from build123d import *

# Parameters (mm, degrees)
SKETCH097_R   = 2.6035
EXTRUDE_DEPTH = 195.262


with BuildPart() as part:
    # Sketch097 → Extrude (new body)
    with BuildSketch(Plane.XY):
        with BuildLine():
            ThreePointArc((12.7, 6.333084), (12.192, 5.825084), (12.7, 5.317084))
            Line((12.7, 4.287469), (12.7, 5.317084))
            ThreePointArc((11.650988, 3.238457), (12.392751, 3.545706), (12.7, 4.287469))
            Line((11.539212, 3.238457), (11.650988, 3.238457))
            ThreePointArc((10.4902, 4.287469), (10.797449, 3.545706), (11.539212, 3.238457))
            Line((10.4902, 6.402089), (10.4902, 4.287469))
            ThreePointArc((10.4902, 6.402089), (9.856505, 7.351068), (8.737131, 7.129409))
            Line((5.441006, 3.840816), (8.737131, 7.129409))
            ThreePointArc((5.441006, 3.840816), (4.750878, 2.809883), (4.5085, 1.593186))
            Line((4.5085, -1.593186), (4.5085, 1.593186))
            ThreePointArc((4.5085, -1.593186), (4.750878, -2.809883), (5.441006, -3.840816))
            Line((8.737131, -7.129409), (5.441006, -3.840816))
            ThreePointArc((8.737131, -7.129409), (9.856505, -7.351068), (10.4902, -6.402089))
            Line((10.4902, -4.287469), (10.4902, -6.402089))
            ThreePointArc((11.539212, -3.238457), (10.797449, -3.545706), (10.4902, -4.287469))
            Line((11.650988, -3.238457), (11.539212, -3.238457))
            ThreePointArc((12.7, -4.287469), (12.392751, -3.545706), (11.650988, -3.238457))
            Line((12.7, -5.317084), (12.7, -4.287469))
            ThreePointArc((12.7, -5.317084), (12.192, -5.825084), (12.7, -6.333084))
            Line((12.7, -9.5504), (12.7, -6.333084))
            ThreePointArc((12.7, -9.5504), (12.192, -10.058323), (12.699847, -10.5664))
            ThreePointArc((10.566443, -12.699848), (12.082538, -12.082507), (12.699847, -10.5664))
            ThreePointArc((10.566443, -12.699848), (10.058367, -12.192), (9.550443, -12.7))
            Line((6.333127, -12.7), (9.550443, -12.7))
            ThreePointArc((6.333127, -12.7), (5.825127, -12.192), (5.317127, -12.7))
            Line((4.287512, -12.7), (5.317127, -12.7))
            ThreePointArc((3.2385, -11.650988), (3.545749, -12.392751), (4.287512, -12.7))
            Line((3.2385, -11.539212), (3.2385, -11.650988))
            ThreePointArc((4.287512, -10.4902), (3.545749, -10.797449), (3.2385, -11.539212))
            Line((6.416408, -10.4902), (4.287512, -10.4902))
            ThreePointArc((6.416408, -10.4902), (7.414731, -9.822813), (7.17965, -8.645193))
            Line((3.95227, -5.42369), (7.17965, -8.645193))
            ThreePointArc((3.95227, -5.42369), (2.922936, -4.736929), (1.709254, -4.4958))
            Line((-1.709254, -4.4958), (1.709254, -4.4958))
            ThreePointArc((-1.709254, -4.4958), (-2.922936, -4.736929), (-3.95227, -5.42369))
            Line((-7.17965, -8.645193), (-3.95227, -5.42369))
            ThreePointArc((-7.17965, -8.645193), (-7.414731, -9.822813), (-6.416408, -10.4902))
            Line((-4.287512, -10.4902), (-6.416408, -10.4902))
            ThreePointArc((-3.2385, -11.539212), (-3.545749, -10.797449), (-4.287512, -10.4902))
            Line((-3.2385, -11.650988), (-3.2385, -11.539212))
            ThreePointArc((-4.287512, -12.7), (-3.545749, -12.392751), (-3.2385, -11.650988))
            Line((-5.317127, -12.7), (-4.287512, -12.7))
            ThreePointArc((-5.317127, -12.7), (-5.825127, -12.192), (-6.333127, -12.7))
            Line((-9.550443, -12.7), (-6.333127, -12.7))
            ThreePointArc((-9.550443, -12.7), (-10.058367, -12.192), (-10.566443, -12.699848))
            ThreePointArc((-12.699847, -10.5664), (-12.082538, -12.082507), (-10.566443, -12.699848))
            ThreePointArc((-12.699847, -10.5664), (-12.192, -10.058323), (-12.7, -9.5504))
            Line((-12.7, -6.333084), (-12.7, -9.5504))
            ThreePointArc((-12.7, -6.333084), (-12.192, -5.825084), (-12.7, -5.317084))
            Line((-12.7, -4.287469), (-12.7, -5.317084))
            ThreePointArc((-11.650988, -3.238457), (-12.392751, -3.545706), (-12.7, -4.287469))
            Line((-11.539212, -3.238457), (-11.650988, -3.238457))
            ThreePointArc((-10.4902, -4.287469), (-10.797449, -3.545706), (-11.539212, -3.238457))
            Line((-10.4902, -6.402089), (-10.4902, -4.287469))
            ThreePointArc((-10.4902, -6.402089), (-9.856505, -7.351068), (-8.737131, -7.129409))
            Line((-5.441006, -3.840816), (-8.737131, -7.129409))
            ThreePointArc((-5.441006, -3.840816), (-4.750878, -2.809883), (-4.5085, -1.593186))
            Line((-4.5085, 1.593186), (-4.5085, -1.593186))
            ThreePointArc((-4.5085, 1.593186), (-4.750878, 2.809883), (-5.441006, 3.840816))
            Line((-8.737131, 7.129409), (-5.441006, 3.840816))
            ThreePointArc((-8.737131, 7.129409), (-9.856505, 7.351068), (-10.4902, 6.402089))
            Line((-10.4902, 4.287469), (-10.4902, 6.402089))
            ThreePointArc((-11.539212, 3.238457), (-10.797449, 3.545706), (-10.4902, 4.287469))
            Line((-11.650988, 3.238457), (-11.539212, 3.238457))
            ThreePointArc((-12.7, 4.287469), (-12.392751, 3.545706), (-11.650988, 3.238457))
            Line((-12.7, 5.317084), (-12.7, 4.287469))
            ThreePointArc((-12.7, 5.317084), (-12.192, 5.825084), (-12.7, 6.333084))
            Line((-12.7, 9.5504), (-12.7, 6.333084))
            ThreePointArc((-12.7, 9.5504), (-12.192, 10.058323), (-12.699847, 10.5664))
            ThreePointArc((-10.566443, 12.699848), (-12.082538, 12.082507), (-12.699847, 10.5664))
            ThreePointArc((-10.566443, 12.699848), (-10.058367, 12.192), (-9.550443, 12.7))
            Line((-6.333127, 12.7), (-9.550443, 12.7))
            ThreePointArc((-6.333127, 12.7), (-5.825127, 12.192), (-5.317127, 12.7))
            Line((-4.287512, 12.7), (-5.317127, 12.7))
            ThreePointArc((-3.2385, 11.650988), (-3.545749, 12.392751), (-4.287512, 12.7))
            Line((-3.2385, 11.539212), (-3.2385, 11.650988))
            ThreePointArc((-4.287512, 10.4902), (-3.545749, 10.797449), (-3.2385, 11.539212))
            Line((-6.476789, 10.4902), (-4.287512, 10.4902))
            ThreePointArc((-6.476789, 10.4902), (-7.432222, 9.851404), (-7.207036, 8.724371))
            Line((-3.898273, 5.423169), (-7.207036, 8.724371))
            ThreePointArc((-3.898273, 5.423169), (-2.86912, 4.736788), (-1.655778, 4.4958))
            Line((1.655778, 4.4958), (-1.655778, 4.4958))
            ThreePointArc((1.655778, 4.4958), (2.86912, 4.736788), (3.898273, 5.423169))
            Line((7.207036, 8.724371), (3.898273, 5.423169))
            ThreePointArc((7.207036, 8.724371), (7.432222, 9.851404), (6.476789, 10.4902))
            Line((4.287512, 10.4902), (6.476789, 10.4902))
            ThreePointArc((3.2385, 11.539212), (3.545749, 10.797449), (4.287512, 10.4902))
            Line((3.2385, 11.650988), (3.2385, 11.539212))
            ThreePointArc((4.287512, 12.7), (3.545749, 12.392751), (3.2385, 11.650988))
            Line((5.317127, 12.7), (4.287512, 12.7))
            ThreePointArc((5.317127, 12.7), (5.825127, 12.192), (6.333127, 12.7))
            Line((9.550443, 12.7), (6.333127, 12.7))
            ThreePointArc((9.550443, 12.7), (10.058367, 12.192), (10.566443, 12.699848))
            ThreePointArc((12.699847, 10.5664), (12.082538, 12.082507), (10.566443, 12.699848))
            ThreePointArc((12.699847, 10.5664), (12.192, 10.058323), (12.7, 9.5504))
            Line((12.7, 6.333084), (12.7, 9.5504))
        make_face()
        Circle(SKETCH097_R, mode=Mode.SUBTRACT)
    extrude(amount=EXTRUDE_DEPTH)


solid = part.part
For this review, take the finished solid that the model builds, in its own axes (mm). A direction names the side the tool comes from. Coordinates: 2 decimals unless noted, no trailing zeros. Order: outer loops, then holes, each group sorted by start corner. A loop starts at its lowest first (then second) coordinate and runs counter-clockwise, first axis right, second up. Notation, with made-up numbers: (-7, -2.75) - (52, -2.75) arc R26 ccw to (52, 22.25) - close; hole circle Ø1 at (25, 60.5). An arc over 180 degrees is marked (long way). Answer as CSV lines item,"result". Start each with the question number.
1) Machinability: for faces 1 (the flat face through (0, -4.496, 96)), 2 (the flat face through (-8, 12.7, 96)), 3 (the flat face through (3, 0, 0)), 4 (the flat face through (-4.508, 0, 96)), 5 (the flat face through (-5.59, -7.06, 96.26)), which of the approach directions +Z, -Z, +X, -X, +Y, -Y give a long, thin tool a straight path to every point of the face, cutting with its end or side? Answer none if there is none.
2) To check wall thickness, follow line 1 along Y through (x, z) = (8.75, 78.5); line 2 along Y through (x, z) = (0, 48.5); line 3 along Y through (x, z) = (6, 131.5). State the ranges of each line that lie inside material, in increasing order. Write a range as [from, to].
3) Draft analysis for pull direction Y (two halves, no side actions). For faces 6 (the cylindrical face through (2.483, 0.782, 96.264)), 7 (the flat face through (-12.7, -8, 96)), 8 (the flat face through (0, 4.496, 96)), state which applies: +Y half, -Y half, draft (parallel to the pull), parting line (faces both ways), or undercut.
4) Add section A-A (x = 0). State the section outline as (y, z) points, then the cut area to 3 significant figures.
5) Add section B-B (y = 0). State the section outline as (x, z) points.
6) Insertion check: P1, Ø3.5, axis at y = -0.5, z = 94, coming from the -X side; P2, Ø2.5, axis at x = -5.5, z = 69, coming from the -Y side; P3, Ø5, axis at x = 1, z = 104.5, coming from the +Y side; P4, Ø1, axis at x = 0, z = 117.5, coming from the -Y side. Each pin has a flat end and moves straight along its axis. Give the tip position at first contact, or say it passes through.
Result:
1,face 1,"+Z, -Z, -Y"
1,face 2,"+Z, -Z, +X, -X, +Y"
1,face 3,"-Z, +X, -X, +Y, -Y"
1,face 4,"+Z, -Z, -X"
1,face 5,"+Z, -Z"
2,line 1,"[-12.7, -7.14], [7.14, 12.7]"
2,line 2,"[-4.5, -2.6], [2.6, 4.5]"
2,line 3,"[-12.22, -10.49], [-7.47, -4.4], [4.4, 7.52], [10.49, 12.22]"
3,face 6,"undercut"
3,face 7,"draft"
3,face 8,"+Y half"
4,outline,"(-4.5, 0) - (-2.6, 0) - (-2.6, 195.26) - (-4.5, 195.26) - close; (2.6, 0) - (4.5, 0) - (4.5, 195.26) - (2.6, 195.26) - close"
4,area,"739 mm^2"
5,outline,"(-4.51, 0) - (-2.6, 0) - (-2.6, 195.26) - (-4.51, 195.26) - close; (2.6, 0) - (4.51, 0) - (4.51, 195.26) - (2.6, 195.26) - close"
6,P1,"x = -4.58"
6,P2,"y = -12.7"
6,P3,"y = 12.34"
6,P4,"y = -4.5"
